Design review of the part built by this model. Coordinates are the model's own, in mm. A direction names the side the tool comes from. Coordinates: 2 decimals unless noted, no trailing zeros. Loops run counter-clockwise (first coordinate to the right, second up) from the corner with the lowest first, then second, coordinate; pieces in that order, holes last. Notation, with made-up numbers: M -13.75,1.5 L 16.25,1.5 A16 ccw 16.25,6.5 Z; hole C 30.5,34 d2. An arc over 180 degrees is marked long. Put each result on its own line as item: value. Start each with the question number.
(1) Take a section at B-B, the plane y = -4.75. Give the boundary of the cut face in (x, z).
(2) For faces 1 (the flat face through (0.2, -8, -4)), 2 (the flat face through (2, 0, -5)), 3 (the flat face through (-4, 3, 0)), 4 (the flat face through (4, 3, 0)), list the 3-axis set-ups (+Z, -Z, +X, -X, +Y, -Y) from which the entire face can be reached by the end or side of a thin tool; tool diameter is ignored.
(3) Take a section at C-C, the plane y = 4.25. Give the boundary of the cut face in (x, z), then the cut area to 3 significant figures.
(4) The part is to be moulded in two halves that separate along X. For faces 5 (the flat face through (0, 6, 0)), 6 (the conical face through (9.61, 2.19, 0.2)), 7 (the flat face through (-0.2, -8, 4)), 8 (the flat face through (-0.74, 4.96, -0.14)), say which applies: +X half, -X half, draft (parallel to the pull), parting line (faces both ways), or undercut.
(5) For probe 1 along Y at (x, z) = (-5.5, 6); probe 2 along Y at (x, z) = (-2.25, 2.25); probe 3 along Z at (x, y) = (-2.75, -3), list the stretches that pass through material, from the lowest coordinate up. Write a range as [from, to].
(6) Clearance check with flat-ended pins moving along their axes: pin 1 (1.6 mm diameter, centred on y = -8, z = -3.5, fed in from +X); pin 2 (4 mm diameter, centred on x = 4.5, y = -3, fed in from +Z); pin 3 (1.5 mm diameter, centred on y = -5.5, z = 4, fed in from +X). State where each tip first meets the part, or that it passes through.
```python
from build123d import *
from build123d.topology import SkipClean

# Parameters (mm, degrees)
ESBO_O2_R                = 10
RESSALTO_EXTRUS_O1_DEPTH = 3
RESSALTO_EXTRUS_O1_TAPER = 10
RESSALTO_EXTRUS_O2_DEPTH = 6
RESSALTO_EXTRUS_O2_DRAFT = 3
RESSALTO_EXTRUS_O3_DEPTH = 6
RESSALTO_EXTRUS_O4_DEPTH = 10


with BuildPart() as part:
    # Esbo_o2 → Ressalto-extrus_o1 (new body)
    with BuildSketch(Plane(origin=(0, 0, 0), x_dir=(1, 0, 0), z_dir=(0, 1, 0))):
        Circle(ESBO_O2_R)
    extrude(amount=RESSALTO_EXTRUS_O1_DEPTH, taper=RESSALTO_EXTRUS_O1_TAPER)


with BuildPart() as ressalto_extrus_o2_tool:
    # Esbo_o2_3 → Ressalto-extrus_o2 (with draft: the straight prism first)
    with BuildSketch(Plane(origin=(0, 0, 0), x_dir=(1, 0, 0), z_dir=(0, 1, 0))):
        with BuildLine():
            Line((-1, 9.949874371), (-1, -9.949874371))
            ThreePointArc((-1, -9.949874371), (0, -10), (1, -9.949874371))
            Line((1, -9.949874371), (1, 9.949874371))
            ThreePointArc((1, 9.949874371), (0, 10), (-1, 9.949874371))
        make_face()
    extrude(amount=RESSALTO_EXTRUS_O2_DEPTH)
    # Ressalto-extrus_o2: the draft: its side faces are tilted about the plane it starts from
    ressalto_extrus_o2_sides = [ressalto_extrus_o2_tool.faces().sort_by_distance(p)[0] for p in [
        (1, 3, 0),
        (0, 3, -10),
        (-1, 3, 0),
        (0, 3, 10),
    ]]
    draft(ressalto_extrus_o2_sides, Plane(origin=(0, 0, 0), x_dir=(1, 0, 0), z_dir=(0, 1, 0)), RESSALTO_EXTRUS_O2_DRAFT)


with BuildPart() as part_1:
    add(part.part)

    # Ressalto-extrus_o2: add ressalto_extrus_o2_tool
    add(ressalto_extrus_o2_tool.part)

    # Esbo_o3 → Ressalto-extrus_o3 (add)
    with BuildSketch(Plane(origin=(0, 0, 0), x_dir=(1, 0, 0), z_dir=(0, 1, 0))):
        with BuildLine():
            Line((-0.2, 2.993325909), (-0.2, 4.995998399))
            ThreePointArc((-0.2, 4.995998399), (-5, 0), (-0.2, -4.995998399))
            Line((-0.2, -4.995998399), (-0.2, -2.993325909))
            ThreePointArc((-0.2, -2.993325909), (-3, 0), (-0.2, 2.993325909))
        make_face()
        with BuildLine():
            ThreePointArc((5, 0), (3.605551275, 3.464101615), (0.2, 4.995998399))
            Line((0.2, 4.995998399), (0.2, 2.993325909))
            ThreePointArc((0.2, 2.993325909), (2.19089023, 2.049390153), (3, 0))
            ThreePointArc((3, 0), (2.19089023, -2.049390153), (0.2, -2.993325909))
            Line((0.2, -2.993325909), (0.2, -4.995998399))
            ThreePointArc((0.2, -4.995998399), (3.605551275, -3.464101615), (5, 0))
        make_face()
        with BuildLine():
            ThreePointArc((0.2, 4.995998399), (0, 5), (-0.2, 4.995998399))
            Line((-0.2, 4.995998399), (-0.2, 2.993325909))
            ThreePointArc((-0.2, 2.993325909), (0, 3), (0.2, 2.993325909))
            Line((0.2, 2.993325909), (0.2, 4.995998399))
        make_face()
        with BuildLine():
            Line((-0.2, -2.993325909), (-0.2, -4.995998399))
            ThreePointArc((-0.2, -4.995998399), (0, -5), (0.2, -4.995998399))
            Line((0.2, -4.995998399), (0.2, -2.993325909))
            ThreePointArc((0.2, -2.993325909), (0, -3), (-0.2, -2.993325909))
        make_face()
    extrude(amount=-RESSALTO_EXTRUS_O3_DEPTH)

    # Esbo_o3_3 → Ressalto-extrus_o4 (add)
    with SkipClean():  # the faces are left unmerged after this step: merging them gives an invalid solid
        with BuildSketch(Plane(origin=(0, 0, 0), x_dir=(1, 0, 0), z_dir=(0, 1, 0))):
            with BuildLine():
                ThreePointArc((5, 0), (3.605551275, 3.464101615), (0.2, 4.995998399))
                Line((0.2, 4.995998399), (0.2, 2.993325909))
                ThreePointArc((0.2, 2.993325909), (2.19089023, 2.049390153), (3, 0))
                ThreePointArc((3, 0), (2.19089023, -2.049390153), (0.2, -2.993325909))
                Line((0.2, -2.993325909), (0.2, -4.995998399))
                ThreePointArc((0.2, -4.995998399), (3.605551275, -3.464101615), (5, 0))
            make_face()
            with BuildLine():
                Line((-0.2, 2.993325909), (-0.2, 4.995998399))
                ThreePointArc((-0.2, 4.995998399), (-5, 0), (-0.2, -4.995998399))
                Line((-0.2, -4.995998399), (-0.2, -2.993325909))
                ThreePointArc((-0.2, -2.993325909), (-3, 0), (-0.2, 2.993325909))
            make_face()
        extrude(amount=-RESSALTO_EXTRUS_O4_DEPTH)


solid = part_1.part
```
Computed values:
1. outline: C 0,0 d10; hole C 0,0 d6
2. face 1: +Z, -Z, -Y
2. face 2: -Y
2. face 3: +Z, -Z, -X, +Y
2. face 4: +Z, -Z, +X, +Y
3. outline: M -0.78,-9.75 A9.78 ccw 0.78,-9.75 L 0.78,9.75 A9.78 ccw -0.78,9.75 Z
3. area: 30.4 mm^2
4. face 5: draft
4. face 6: +X half
4. face 7: undercut
4. face 8: -X half
5. probe 1: y = [0, 3]
5. probe 2: y = [-10, 3]
5. probe 3: z = [-4.18, -1.2], [1.2, 4.18]
6. pin 1: stops at x = 4.21
6. pin 2: stops at z = 4.33
6. pin 3: stops at x = 3.8
